Model file for the job. Use its own axes, mm. Face numbers are marked on the shaded views. Coordinates: 2 decimals unless noted, no trailing zeros. Order: outer loops, then holes, each group sorted by start corner. A loop starts at its lowest first (then second) coordinate and runs counter-clockwise, first axis right, second up. Notation, with made-up numbers: (21.5, -7) -> (63.5, -7) arc R22 ccw to (63.5, 32) -> close; hole circle Ø2 at (74, 53.25). An arc over 180 degrees is marked (long way). Return JSON: item names as keys, results as strings. Group by question number.
1) Cut at D-D (y = -102). Write the cut outline in (x, z) (3 decimals).
2) Pull direction Y, two halves, no side cores. Call the marked faces 1 and 2: +Y half, -Y half, draft (parallel to the pull), parting line (faces both ways), or undercut.
3) Flat gauge pins, fed straight in: pin 1 (1 mm diameter, centred on x = 102, z = 45.5, fed in from +Y); pin 2 (2 mm diameter, centred on x = 97.5, y = -97.5, fed in from -Z); pin 3 (6.5 mm diameter, centred on y = 92, z = 20.5, fed in from -X). Where does each tip first touch, or does it go through?
4) Cut at B-B (z = 17). Write the cut outline in (x, y), and give its area (3 significant figures).
5) Cut at A-A (y = -28.4). Write the cut outline in (x, z).
6) Cut at C-C (z = 34.45). Write the cut outline in (x, y), and give its area (3 significant figures).
7) Probe line 1 (Y direction, x = 102.8, z = 17); line 2 (Y direction, x = 99, z = 17.5); line 3 (Y direction, x = 100.45, z = 17). List the from-to ranges inside material, lowest first.
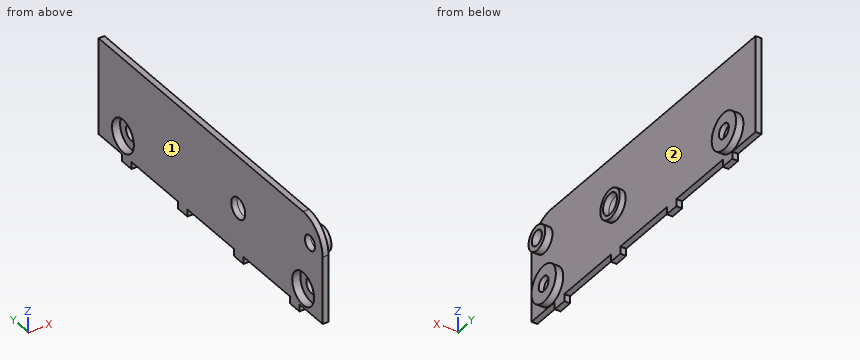
from build123d import *

# Parameters (mm, degrees)
SKETCH1_W            = 200
SKETCH1_H            = 230
BOSS_EXTRUDE1_DEPTH  = 70
SKETCH2_W            = 192
SKETCH2_H            = 222
CUT_EXTRUDE1_DEPTH   = 66
SKETCH4_W            = 196
SKETCH4_H            = 25
CUT_EXTRUDE3_DEPTH   = 10
SKETCH10_R           = 5
CUT_EXTRUDE8_DEPTH   = 167.075284133
SKETCH11_W           = 2
SKETCH11_H           = 10
BOSS_EXTRUDE2_DEPTH  = 20
SKETCH12_W           = 2
SKETCH12_H           = 5
CUT_EXTRUDE9_DEPTH   = 20
FILLET1_R            = 2.5
SKETCH13_W           = 2
SKETCH13_H           = 10
BOSS_EXTRUDE3_DEPTH  = 20
SKETCH14_W           = 2
SKETCH14_H           = 5
CUT_EXTRUDE10_DEPTH  = 20
FILLET2_R            = 2.5
SKETCH15_W           = 192
SKETCH15_H           = 66
CUT_EXTRUDE11_DEPTH  = 267.458251889
BOSS_EXTRUDE4_DEPTH  = 2
SKETCH18_R           = 7.15
CUT_EXTRUDE12_DEPTH  = 248.638849941
SKETCH19_R           = 5.05
CUT_EXTRUDE13_DEPTH  = 248.638849941
SKETCH20_R           = 5.05
CUT_EXTRUDE14_DEPTH  = 248.638849941
BOSS_EXTRUDE5_START  = 2
BOSS_EXTRUDE5_DEPTH  = 2
SKETCH21_W           = 20
SKETCH21_H           = 10
CUT_EXTRUDE15_DEPTH  = 248.638849941
SKETCH22_W           = 92
SKETCH22_H           = 40
CUT_EXTRUDE16_DEPTH  = 10
SKETCH24_R           = 5.15
CUT_EXTRUDE18_DEPTH  = 242.091269025
FILLET3_R            = 20
FILLET4_R            = 20
SKETCH25_W           = 200
SKETCH25_H           = 4.119110625
CUT_EXTRUDE19_DEPTH  = 261.384331326
SKETCH26_W           = 4
SKETCH26_H           = 65.880889375
CUT_EXTRUDE20_DEPTH  = 261.384331326
SKETCH27_W           = 4
SKETCH27_H           = 9.8
BOSS_EXTRUDE6_DEPTH  = 4.9
SKETCH28_W           = 4
SKETCH28_H           = 9.8
BOSS_EXTRUDE7_DEPTH  = 4.9
SKETCH29_R           = 12.5
SKETCH29_R_2         = 5.05
BOSS_EXTRUDE8_DEPTH  = 9
SKETCH30_R           = 8.5
SKETCH30_R_2         = 5.15
BOSS_EXTRUDE9_DEPTH  = 5
SKETCH32_R           = 10
SKETCH32_R_2         = 7.15
BOSS_EXTRUDE10_DEPTH = 4
SKETCH33_R           = 11.2
CUT_EXTRUDE21_DEPTH  = 5.5


with BuildPart() as part:
    # Sketch1 → Boss-Extrude1 (new body)
    with BuildSketch(Plane.XY):
        Rectangle(SKETCH1_W, SKETCH1_H)
    extrude(amount=BOSS_EXTRUDE1_DEPTH)

    # Sketch2 → Cut-Extrude1 (cut)
    with BuildSketch(Plane.XY.offset(70)):
        Rectangle(SKETCH2_W, SKETCH2_H)
    extrude(amount=-CUT_EXTRUDE1_DEPTH, mode=Mode.SUBTRACT)

    # Sketch4 → Cut-Extrude3 (cut)
    with BuildSketch(Plane.XZ.offset(115)):
        with Locations((0, 57.5)):
            Rectangle(SKETCH4_W, SKETCH4_H)
    extrude(amount=-CUT_EXTRUDE3_DEPTH, mode=Mode.SUBTRACT)

    # Sketch10 → Cut-Extrude8 (cut, through all)
    with BuildSketch(Plane.XY.offset(4)):
        with Locations((0, -11)):
            Circle(SKETCH10_R)
    extrude(amount=-CUT_EXTRUDE8_DEPTH, mode=Mode.SUBTRACT)

    # Sketch11 → Boss-Extrude2 (add)
    with BuildSketch(Plane.XY.offset(70)):
        with Locations((-99, -110)):
            Rectangle(SKETCH11_W, SKETCH11_H)
    extrude(amount=BOSS_EXTRUDE2_DEPTH)

    # Sketch12 → Cut-Extrude9 (cut)
    with BuildSketch(Plane.XY.offset(90)):
        with Locations((-99, -110)):
            Rectangle(SKETCH12_W, SKETCH12_H)
    extrude(amount=-CUT_EXTRUDE9_DEPTH, mode=Mode.SUBTRACT)

    # Fillet1
    fillet1_edges = [part.edges().sort_by_distance(p)[0] for p in [
        (-99, -112.5, 70),
        (-99, -107.5, 70),
    ]]
    fillet(fillet1_edges, radius=FILLET1_R - 0.0001)  # a hair under: the kernel refuses the full size

    # Sketch13 → Boss-Extrude3 (add)
    with BuildSketch(Plane.XY.offset(70)):
        with Locations((99, -110)):
            Rectangle(SKETCH13_W, SKETCH13_H)
    extrude(amount=BOSS_EXTRUDE3_DEPTH)

    # Sketch14 → Cut-Extrude10 (cut)
    with BuildSketch(Plane.XY.offset(90)):
        with Locations((99, -110)):
            Rectangle(SKETCH14_W, SKETCH14_H)
    extrude(amount=-CUT_EXTRUDE10_DEPTH, mode=Mode.SUBTRACT)

    # Fillet2
    fillet2_edges = [part.edges().sort_by_distance(p)[0] for p in [
        (99, -112.5, 70),
        (99, -107.5, 70),
    ]]
    fillet(fillet2_edges, radius=FILLET2_R - 0.0001)  # a hair under: the kernel refuses the full size

    # Sketch15 → Cut-Extrude11 (cut, through all)
    with BuildSketch(Plane(origin=(0, 115, 0), x_dir=(1, 0, 0), z_dir=(0, 1, 0))):
        with Locations((0, -37)):
            Rectangle(SKETCH15_W, SKETCH15_H)
    extrude(amount=-CUT_EXTRUDE11_DEPTH, mode=Mode.SUBTRACT)

    # Sketch16 → Boss-Extrude4 (add)
    with BuildSketch(Plane(origin=(-98, 0, 0), x_dir=(0, 0, -1), z_dir=(1, 0, 0))):
        with BuildLine():
            Line((-90, -107.5), (-72.5, -107.5))
            ThreePointArc((-72.5, -107.5), (-70, -110), (-72.5, -112.5))
            Line((-72.5, -112.5), (-90, -112.5))
            Line((-90, -112.5), (-90, -115))
            Line((-90, -115), (-45, -115))
            Line((-45, -115), (-45, -105))
            Line((-45, -105), (-90, -105))
            Line((-90, -105), (-90, -107.5))
        make_face()
    extrude(amount=BOSS_EXTRUDE4_DEPTH)

    # Sketch18 → Cut-Extrude12 (cut, through all)
    with BuildSketch(Plane(origin=(100, 0, 0), x_dir=(0, 0, -1), z_dir=(1, 0, 0))):
        with Locations((-34.45, -28.4)):
            Circle(SKETCH18_R)
    extrude(amount=-CUT_EXTRUDE12_DEPTH, mode=Mode.SUBTRACT)

    # Sketch19 → Cut-Extrude13 (cut, through all)
    with BuildSketch(Plane(origin=(100, 0, 0), x_dir=(0, 0, -1), z_dir=(1, 0, 0))):
        with Locations((-17, -95)):
            Circle(SKETCH19_R)
    extrude(amount=-CUT_EXTRUDE13_DEPTH, mode=Mode.SUBTRACT)

    # Sketch20 → Cut-Extrude14 (cut, through all)
    with BuildSketch(Plane(origin=(100, 0, 0), x_dir=(0, 0, -1), z_dir=(1, 0, 0))):
        with Locations((-17, 90)):
            Circle(SKETCH20_R)
    extrude(amount=-CUT_EXTRUDE14_DEPTH, mode=Mode.SUBTRACT)

    # Sketch17 → Boss-Extrude5 (add)
    with BuildSketch(Plane.ZY.offset(-98).offset(BOSS_EXTRUDE5_START)):
        with BuildLine():
            Line((90, -107.5), (72.5, -107.5))
            ThreePointArc((72.5, -107.5), (70, -110), (72.5, -112.5))
            Line((72.5, -112.5), (90, -112.5))
            Line((90, -112.5), (90, -115))
            Line((90, -115), (45, -115))
            Line((45, -115), (45, -105))
            Line((45, -105), (90, -105))
            Line((90, -105), (90, -107.5))
        make_face()
    extrude(amount=-BOSS_EXTRUDE5_DEPTH)

    # Sketch21 → Cut-Extrude15 (cut, through all)
    with BuildSketch(Plane(origin=(100, 0, 0), x_dir=(0, 0, -1), z_dir=(1, 0, 0))):
        with Locations((-80, -110)):
            Rectangle(SKETCH21_W, SKETCH21_H)
    extrude(amount=-CUT_EXTRUDE15_DEPTH, mode=Mode.SUBTRACT)

    # Sketch22 → Cut-Extrude16 (cut)
    with BuildSketch(Plane.XY.offset(4)):
        with Locations((0, 95)):
            Rectangle(SKETCH22_W, SKETCH22_H)
    extrude(amount=-CUT_EXTRUDE16_DEPTH, mode=Mode.SUBTRACT)

    # Sketch24 → Cut-Extrude18 (cut, through all)
    with BuildSketch(Plane(origin=(100, 0, 0), x_dir=(0, 0, -1), z_dir=(1, 0, 0))):
        with Locations((-52.45, -102)):
            Circle(SKETCH24_R)
    extrude(amount=-CUT_EXTRUDE18_DEPTH, mode=Mode.SUBTRACT)

    # Fillet3
    fillet3_edges = [part.edges().sort_by_distance(p)[0] for p in [
        (98, -115, 70),
    ]]
    fillet(fillet3_edges, radius=FILLET3_R)

    # Fillet4
    fillet4_edges = [part.edges().sort_by_distance(p)[0] for p in [
        (-98, -115, 70),
    ]]
    fillet(fillet4_edges, radius=FILLET4_R)

    # Sketch25 → Cut-Extrude19 (cut, through all)
    with BuildSketch(Plane(origin=(0, 115, 0), x_dir=(1, 0, 0), z_dir=(0, 1, 0))):
        with Locations((0, -2.059555313)):
            Rectangle(SKETCH25_W, SKETCH25_H)
    extrude(amount=-CUT_EXTRUDE19_DEPTH, mode=Mode.SUBTRACT)


with BuildPart() as cut_extrude19_piece_1:
    # of the separate pieces the step leaves, piece 1, a body of its own (cut_extrude19_pieces)
    add(part.part.solids().sort_by_distance((100, -115, 4.119110625))[0])

    # Sketch27 → Boss-Extrude6 (add)
    with BuildSketch(Plane(origin=(0, 0, 4.119110625), x_dir=(-1, 0, 0), z_dir=(0, 0, -1))):
        with Locations((-98, -86.25)):
            Rectangle(SKETCH27_W, SKETCH27_H)
    boss_extrude6 = extrude(amount=BOSS_EXTRUDE6_DEPTH)

    # Sketch28 → Boss-Extrude7 (add)
    with BuildSketch(Plane(origin=(0, 0, 4.119110625), x_dir=(-1, 0, 0), z_dir=(0, 0, -1))):
        with Locations((-98, -28.75)):
            Rectangle(SKETCH28_W, SKETCH28_H)
    boss_extrude7 = extrude(amount=BOSS_EXTRUDE7_DEPTH)

    # Mirror1: Boss-Extrude6, Boss-Extrude7 across plane
    add(boss_extrude6.mirror(Plane.ZX))
    add(boss_extrude7.mirror(Plane.ZX))

    # Sketch29 → Boss-Extrude8 (add)
    with BuildSketch(Plane.ZY.offset(-96)):
        with Locations((17, 90)):
            Circle(SKETCH29_R)
        with Locations(Location((17, 90, 0), (0, 0, 180))):
            Circle(SKETCH29_R_2, mode=Mode.SUBTRACT)
    boss_extrude8 = extrude(amount=-BOSS_EXTRUDE8_DEPTH)

    # Sketch30 → Boss-Extrude9 (add)
    with BuildSketch(Plane(origin=(100, 0, 0), x_dir=(0, 0, -1), z_dir=(1, 0, 0))):
        with Locations(Location((-52.45, -102, 0), (0, 0, 180))):
            Circle(SKETCH30_R)
        with Locations((-52.45, -102)):
            Circle(SKETCH30_R_2, mode=Mode.SUBTRACT)
    extrude(amount=BOSS_EXTRUDE9_DEPTH)

    # Sketch32 → Boss-Extrude10 (add)
    with BuildSketch(Plane(origin=(100, 0, 0), x_dir=(0, 0, -1), z_dir=(1, 0, 0))):
        with Locations(Location((-34.45, -28.4, 0), (0, 0, 180))):
            Circle(SKETCH32_R)
        with Locations((-34.45, -28.4)):
            Circle(SKETCH32_R_2, mode=Mode.SUBTRACT)
    extrude(amount=BOSS_EXTRUDE10_DEPTH)

    # Sketch33 → Cut-Extrude21 (cut)
    with BuildSketch(Plane.ZY.offset(-96)):
        with Locations((17, 90)):
            Circle(SKETCH33_R)
    cut_extrude21 = extrude(amount=-CUT_EXTRUDE21_DEPTH, mode=Mode.SUBTRACT)

    # Mirror2: Boss-Extrude8, Cut-Extrude21 across plane
    add(boss_extrude8.mirror(Plane.ZX.offset(-2.5)))
    add(cut_extrude21.mirror(Plane.ZX.offset(-2.5)), mode=Mode.SUBTRACT)


with BuildPart() as cut_extrude19_piece_2:
    # of the separate pieces the step leaves, piece 2, a body of its own (cut_extrude19_pieces)
    add(part.part.solids().sort_by_distance((-100, -115, 50))[0])

    # Sketch26 → Cut-Extrude20 (cut, through all)
    with BuildSketch(Plane(origin=(0, 115, 0), x_dir=(1, 0, 0), z_dir=(0, 1, 0))):
        with Locations((-98, -37.059555313)):
            Rectangle(SKETCH26_W, SKETCH26_H)
    extrude(amount=-CUT_EXTRUDE20_DEPTH, mode=Mode.SUBTRACT)


solid = cut_extrude19_piece_1.part
Answers below:
{
 "1": {"outline": "(96, 4.119) -> (100, 4.119) -> (100, 6.644) -> (105, 6.644) -> (105, 27.356) -> (100, 27.356) -> (100, 43.95) -> (105, 43.95) -> (105, 47.3) -> (96, 47.3) -> (96, 25.743) -> (101.5, 25.743) -> (101.5, 8.257) -> (96, 8.257) -> close; (96, 57.6) -> (105, 57.6) -> (105, 60.95) -> (100, 60.95) -> (100, 68.735) -> (96, 68.735) -> close"},
 "2": {"face 1": "draft", "face 2": "undercut"},
 "3": {"pin 1": "stops at y = -96.46", "pin 2": "stops at z = 4.12", "pin 3": "stops at x = 101.5"},
 "4": {"outline": "(96, -115) -> (100, -115) -> (100, -107.5) -> (105, -107.5) -> (105, -100.05) -> (101.5, -100.05) -> (101.5, -106.2) -> (96, -106.2) -> close; (96, -83.8) -> (101.5, -83.8) -> (101.5, -89.95) -> (105, -89.95) -> (105, -82.5) -> (100, -82.5) -> (100, 77.5) -> (105, 77.5) -> (105, 84.95) -> (101.5, 84.95) -> (101.5, 78.8) -> (96, 78.8) -> close; (96, 101.2) -> (101.5, 101.2) -> (101.5, 95.05) -> (105, 95.05) -> (105, 102.5) -> (100, 102.5) -> (100, 115) -> (96, 115) -> close", "area": "853 mm^2"},
 "5": {"outline": "(96, -0.78) -> (100, -0.78) -> (100, 24.45) -> (104, 24.45) -> (104, 27.3) -> (96, 27.3) -> close; (96, 41.6) -> (104, 41.6) -> (104, 44.45) -> (100, 44.45) -> (100, 70) -> (96, 70) -> close"},
 "6": {"outline": "(96, -115) -> (100, -115) -> (100, -38.4) -> (104, -38.4) -> (104, -35.55) -> (96, -35.55) -> close; (96, -21.25) -> (104, -21.25) -> (104, -18.4) -> (100, -18.4) -> (100, 115) -> (96, 115) -> close", "area": "886 mm^2"},
 "7": {"line 1": "y = -107.5 to -100.05, -89.95 to -82.5, 77.5 to 84.95, 95.05 to 102.5", "line 2": "y = -115 to -106.19, -83.81 to 78.81, 101.19 to 115", "line 3": "y = -107.5 to -106.2, -83.8 to -82.5, 77.5 to 78.8, 101.2 to 102.5"}
}
